Build history of the part. All positions in model axes, mm. Give positions to 0.01 mm unless a question says otherwise; leave off trailing zeros. Order: outer loops, then holes, each group sorted by start corner. A loop starts at its lowest first (then second) coordinate and runs counter-clockwise, first axis right, second up. Notation, with made-up numbers: M 49,58.25 L 96,58.25 A34 cw 96,91.25 Z; hole C 60.5,14 d11. An arc over 180 degrees is marked long. Use CSV: the item, a comma, the result in double quotes. Start each with the question number.
Item 1: Band-saw the part on A-A on y = 0. Write the cut outline in (x, z), plus the area to 3 significant figures.
Item 2: Band-saw the part on C-C on z = 15.25. Write the cut outline in (x, y).
Item 3: Wall check: line 1 along Z through (x, y) = (-2.75, -0.5); line 2 along Y through (x, z) = (0, 19.05); line 3 along X through (y, z) = (3, 9.5). Give the ranges that are in metal, low to high.
Item 4: Pin check, flat tips, straight feed: P1, Ø2, axis at x = 0.5, y = 0, coming from the +Z side; P2, Ø3, axis at y = -2, z = 2, coming from the -X side; P3, Ø3, axis at x = 1.5, y = 2.5, coming from the -Z side; P4, Ø1.5, axis at x = -1.5, z = 14.5, coming from the -Y side. Stop position of each tip, or through.
Item 5: Two-plate mould, pull along X, no slides. Class faces 1 (the cylindrical face through (-0.29, 2.23, 19.75)), 2 (the flat face through (0, 0, 0)), 3 (the cylindrical face through (-3.746, 0.165, 9.614)): pulls with the +X half, pulls with the -X half, needs draft (parallel to the pull), parting line crosses it, or undercut.
from build123d import *

# Parameters (mm, degrees)
SKETCH053_R     = 3.75
PAD026_DEPTH    = 20
SKETCH054_R     = 2.25
POCKET018_DEPTH = 0.5
SKETCH050_R     = 3.25
POCKET016_DEPTH = 1
FILLET007_R     = 0.5


with BuildPart() as part:
    # Sketch053 → Pad026 (new body)
    with BuildSketch(Plane.XY):
        Circle(SKETCH053_R)
    extrude(amount=PAD026_DEPTH)

    # Sketch054 (on Face3 of Pad026) → Pocket018 (cut)
    with BuildSketch(Plane.XY.offset(20)):
        Circle(SKETCH054_R)
    extrude(amount=-POCKET018_DEPTH, mode=Mode.SUBTRACT)

    # Sketch050 (on Face5 of Pocket018) → Pocket016 (cut)
    with BuildSketch(Plane.XY.offset(19.5)):
        Circle(SKETCH050_R)
    extrude(amount=-POCKET016_DEPTH, mode=Mode.SUBTRACT)

    # Fillet007
    fillet007_edges = [part.edges().sort_by_distance(p)[0] for p in [
        (-3.75, 0, 20),
    ]]
    fillet(fillet007_edges, radius=FILLET007_R)


solid = part.part
Model answer:
1,outline,"M -3.75,0 L 3.75,0 L 3.75,19.5 A0.5 ccw 3.25,20 L 2.25,20 L 2.25,19.5 L 3.25,19.5 L 3.25,18.5 L -3.25,18.5 L -3.25,19.5 L -2.25,19.5 L -2.25,20 L -3.25,20 A0.5 ccw -3.75,19.5 Z"
1,area,"141 mm^2"
2,outline,"C 0,0 d7.5"
3,line 1,"z = 0 to 18.5, 19.5 to 20"
3,line 2,"y = -3.75 to -3.25, 3.25 to 3.75"
3,line 3,"x = -2.25 to 2.25"
4,P1,"stops at z = 18.5"
4,P2,"stops at x = -3.72"
4,P3,"stops at z = 0"
4,P4,"stops at y = -3.67"
5,face 1,"undercut"
5,face 2,"needs draft"
5,face 3,"parting line crosses it"
